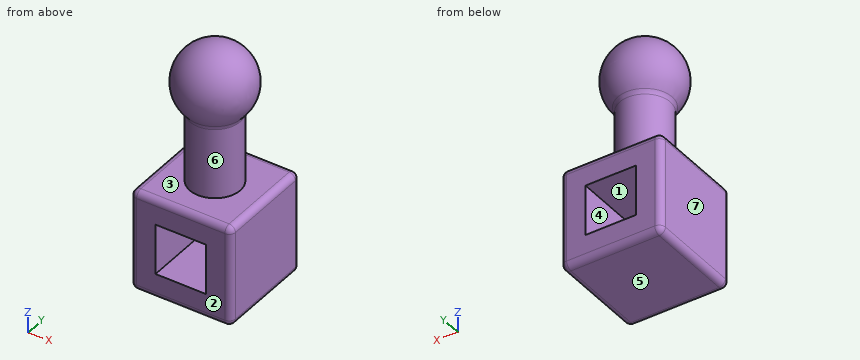
from build123d import *

# Parameters (mm, degrees)
F0_W     = 101.6
F0_H     = 101.6
F1_DEPTH = 101.6
F2_R     = 25.4
F3_DEPTH = 101.6
F6_W     = 50.8
F6_H     = 50.8
F7_DEPTH = 101.6
F8_R     = 6.35


with BuildPart() as f1:
    # F0 (on Top) → F1 (new body)
    with BuildSketch(Plane.XY):
        Rectangle(F0_W, F0_H)
    extrude(amount=F1_DEPTH)

    # F2 (on face) → F3 (join)
    with BuildSketch(Plane.XY.offset(101.6)):
        Circle(F2_R)
    extrude(amount=F3_DEPTH)

    # F4 (on face) → F5 (revolve)
    with BuildSketch(Plane.XY.offset(203.2)):
        with BuildLine():
            Line((0, -25.4), (0, -38.1))
            ThreePointArc((0, -38.1), (38.1, 0), (0, 38.1))
            Line((0, 38.1), (0, 25.4))
            ThreePointArc((0, 25.4), (17.9605122421, 17.9605122421), (25.4, 0))
            ThreePointArc((25.4, 0), (17.9605122421, -17.9605122421), (0, -25.4))
        make_face()
        with BuildLine():
            Line((0, 25.4), (0, -25.4))
            ThreePointArc((0, -25.4), (17.9605122421, -17.9605122421), (25.4, 0))
            ThreePointArc((25.4, 0), (17.9605122421, 17.9605122421), (0, 25.4))
        make_face()
    revolve(axis=Axis((0, 0, 203.2), (0, -1, 0)))

    # F6 (on face) → F7 (cut)
    with BuildSketch(Plane.XZ.offset(50.8)):
        with Locations((0, 50.8)):
            Rectangle(F6_W, F6_H)
    extrude(amount=-F7_DEPTH, mode=Mode.SUBTRACT)

    # F8
    f8_edges = [f1.edges().sort_by_distance(p)[0] for p in [
        (0, 50.8, 101.6),
        (50.8, 0, 101.6),
        (0, -50.8, 101.6),
        (-50.8, 50.8, 50.8),
        (-50.8, -50.8, 50.8),
        (-50.8, 0, 0),
        (-50.8, 0, 101.6),
        (50.8, 50.8, 50.8),
        (0, 50.8, 0),
        (50.8, -50.8, 50.8),
        (0, -50.8, 0),
        (50.8, 0, 0),
        (-25.4, 0, 174.801937),
    ]]
    fillet(f8_edges, radius=F8_R)


solid = f1.part
Read the model definition and answer for the solid it produces. Units are mm, in the model's axes. Face numbers are marked on the shaded views. A direction names the side the tool comes from. Give positions to 0.01 mm unless a question says otherwise; leave off trailing zeros. Loops run counter-clockwise (first coordinate to the right, second up) from the corner with the lowest first, then second, coordinate; pieces in that order, holes last. Notation, with made-up numbers: (-13, -17) - (13, -17) arc R15 ccw to (13, -3) - close; hole circle Ø9 at (-14.5, 45). An arc over 180 degrees is marked (long way). Answer as CSV lines item,"result". Start each with the question number.
1) Find section D-D (z = 154.5). Write down the section's boundary in (x, y).
2) Find section C-C (y = -32.5). Write down the section's boundary in (x, z).
3) Determine the mould class of the marked faces 4, 5, 6 and 7 for opening direction Z: released by +Z, released by -Z, zero draft, split by the parting line, or undercut.
4) Each of these flat-tipped pins is pushed along its axis until it touches: pin 1 Ø2 at (x, y) = (27.5, -3.5) entering from +Z; pin 2 Ø1.5 at (x, z) = (17.5, 132.5) entering from +Y; pin 3 Ø15 at (x, y) = (-9.5, 2) entering from +Z. Where does it stop, or does it pass through?
5) Straight lines are drawn through the part: L1, parallel to X at y = 23.5, z = 61.5; L2, parallel to Z at x = -11, y = 24.5; L3, parallel to Z at x = -24.5, y = -26. For each, find the intervals that lie inside material, in ascending order. Write a range as from..to.
6) Find section B-B (x = -41). Write down the section's boundary in (y, z).
7) Which of the six approach directions +Z, -Z, +X, -X, +Y, -Y give full straight-line access (tool end or side, diameter ignored) to the marked faces 1, 2 and 3?
8) Find section A-A (z = 35). Write down the section's boundary in (x, y).
Findings below:
1,outline,"circle Ø50.8 at (0, 0)"
2,outline,"(-50.8, 6.35) arc R6.35 ccw to (-44.45, 0) - (44.45, 0) arc R6.35 ccw to (50.8, 6.35) - (50.8, 95.25) arc R6.35 ccw to (44.45, 101.6) - (-44.45, 101.6) arc R6.35 ccw to (-50.8, 95.25) - close; circle Ø39.77 at (0, 203.2); hole (-25.4, 25.4) - (25.4, 25.4) - (25.4, 76.2) - (-25.4, 76.2) - close"
3,face 4,"undercut"
3,face 5,"released by -Z"
3,face 6,"undercut"
3,face 7,"zero draft"
4,pin 1,"z = 230.36"
4,pin 2,"y = 19.09"
4,pin 3,"z = 241.24"
5,L1,"-50.8..-25.4, 25.4..50.8"
5,L2,"0..25.4, 76.2..101.6, 176.14..230.23"
5,L3,"0..25.4, 76.2..101.6, 189.96..216.44"
6,outline,"(-50.8, 6.35) arc R6.35 ccw to (-44.45, 0) - (44.45, 0) arc R6.35 ccw to (50.8, 6.35) - (50.8, 95.25) arc R6.35 ccw to (44.45, 101.6) - (-44.45, 101.6) arc R6.35 ccw to (-50.8, 95.25) - close"
7,face 1,"+Y, -Y"
7,face 2,"+Z, -Z, +X, -X, -Y"
7,face 3,"none"
8,outline,"(-50.8, -44.45) arc R6.35 ccw to (-44.45, -50.8) - (-25.4, -50.8) - (-25.4, 50.8) - (-44.45, 50.8) arc R6.35 ccw to (-50.8, 44.45) - close; (25.4, -50.8) - (44.45, -50.8) arc R6.35 ccw to (50.8, -44.45) - (50.8, 44.45) arc R6.35 ccw to (44.45, 50.8) - (25.4, 50.8) - close"
